Geometry: see drawing. Coordinates: mm, zero at the bounding-box minimum. Give positions to 0.01 mm unless a question says otherwise; leave off trailing zeros. Loops run counter-clockwise (first coordinate to the right, second up) from the corner with the lowest first, then second, coordinate; pieces in that order, holes last. Notation, with made-up numbers: (-15.5, 78.5) - (43.5, 78.5) arc R33 cw to (43.5, 108.5) - close; hole circle Ø10 at (29.5, 37). An arc over 180 degrees is marked (long way). One line per question, with ' | ' between items. Start each with the question number.
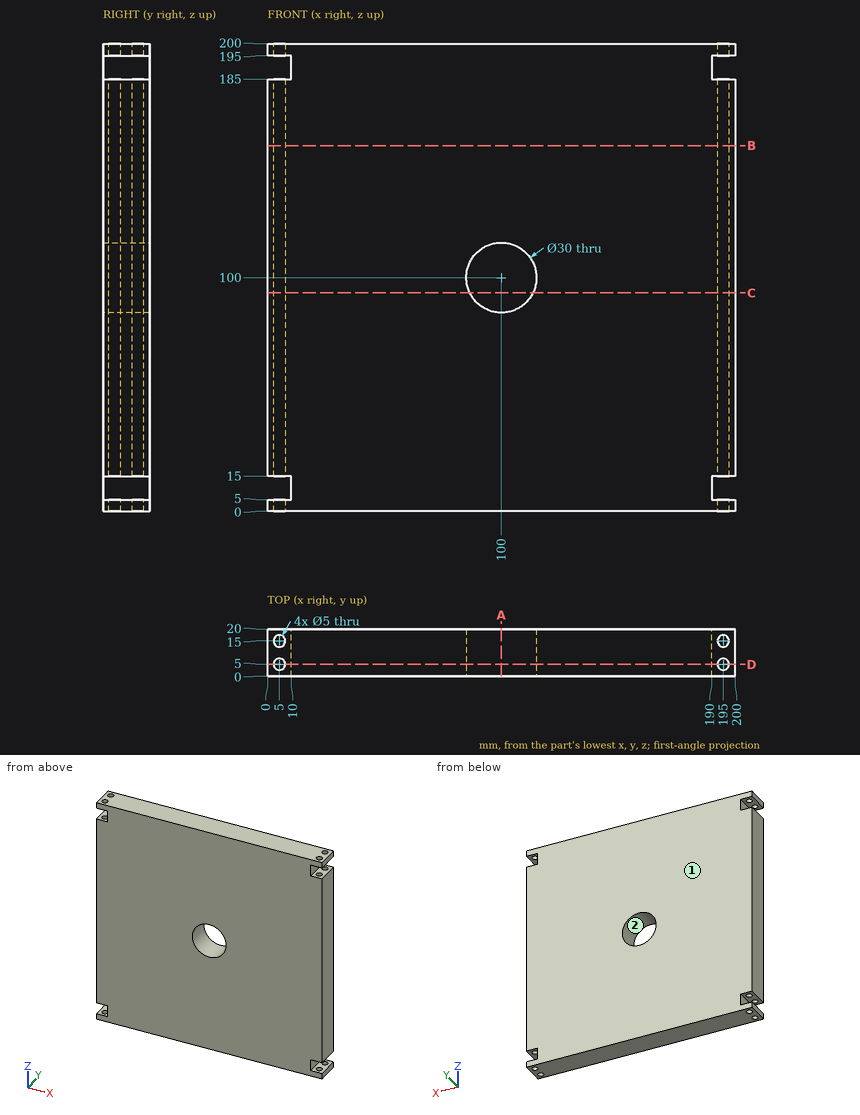
Q1. Section D-D, the plane y = 5. Count the separate pieces of the cut face and the enclosed holes in it, plus the area to 3 significant figures.
Q2. Section A-A, the plane x = 100. Output: boundary loops of the cut face in (y, z), plus the area to 3 significant figures.
Q3. Draft query along X for the marked faces 1 and 2. Return one class per face: +X half, -X half, draft (parallel to the pull), parting line (faces both ways), or undercut.
Q4. Section C-C, the plane z = 93.5. Output: boundary loops of the cut face in (x, y).
Q5. Section B-B, the plane z = 156.5. Output: boundary loops of the cut face in (x, y).
Q6. First-contact query: pin 1 (5 mm diameter, centred on y = 5, z = 188, fed in from -X); pin 2 (8 mm diameter, centred on y = 15, z = 10, fed in from +X). Flat tips, straight axial feed; report the tip coordinate or a pass-through.
Q7. Line query: L1, parallel to X at y = 4.75, z = 61; L2, parallel to Y at x = 195, z = 2.4; L3, parallel to X at y = 4.25, z = 181. Output: solid intervals per line, ascending. Write a range as from..to.
Solved:
1) separate pieces: 7 | enclosed holes: 1 | area: 37,100 mm²
2) outline: (0, 0) - (20, 0) - (20, 85) - (0, 85) - close; (0, 115) - (20, 115) - (20, 200) - (0, 200) - close | area: 3,400 mm²
3) face 1: draft | face 2: undercut
4) outline: (0, 0) - (86.48, 0) - (86.48, 20) - (0, 20) - close; (113.52, 0) - (200, 0) - (200, 20) - (113.52, 20) - close; hole circle Ø5 at (5, 5); hole circle Ø5 at (5, 15); hole circle Ø5 at (195, 5); hole circle Ø5 at (195, 15)
5) outline: (0, 0) - (200, 0) - (200, 20) - (0, 20) - close; hole circle Ø5 at (5, 5); hole circle Ø5 at (5, 15); hole circle Ø5 at (195, 5); hole circle Ø5 at (195, 15)
6) pin 1: stops at x = 10 | pin 2: stops at x = 190
7) L1: x = 0..2.51, 7.49..192.51, 197.49..200 | L2: y = 0..2.5, 7.5..12.5, 17.5..20 | L3: x = 0..2.62, 7.38..192.62, 197.38..200
